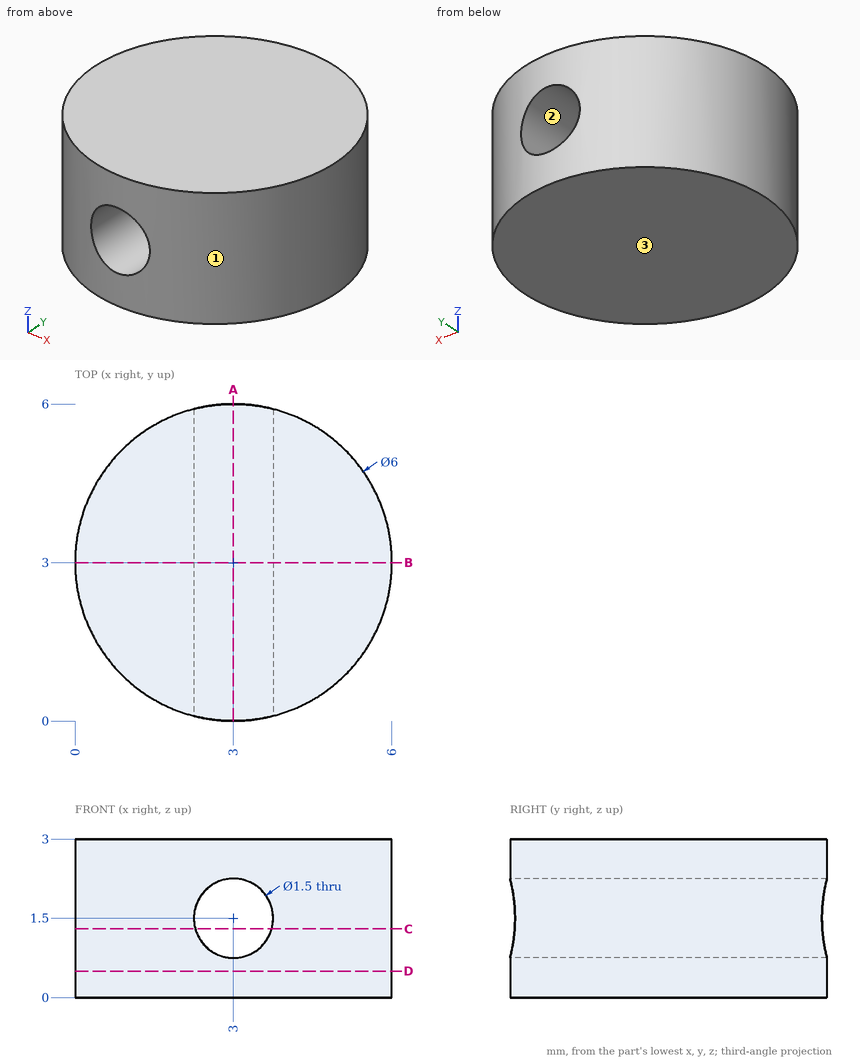
Could you check a few things on this drawing? It's one solid part, dimensions in mm from its lowest x, y, z. Give positions to 0.01 mm unless a question says otherwise; leave off trailing zeros. Order: outer loops, then holes, each group sorted by start corner. A loop starts at its lowest first (then second) coordinate and runs counter-clockwise, first axis right, second up.
1. Suppose I cut it at D-D (z = 0.5). Write out the boundary of the cut face in (x, y), plus the area to 3 significant figures.
Answers below:
outline: circle Ø6 at (3, 3)
area: 28.3 mm2
2. Suppose I cut it at B-B (y = 3). Write out the boundary of the cut face in (x, z).
Answers below:
outline: (0, 0) - (6, 0) - (6, 3) - (0, 3) - close; hole circle Ø1.5 at (3, 1.5)
3. Thinking about a two-plate mould opening in X: for the marked faces 1, 2 and 3, which applies, +X half, -X half, draft (parallel to the pull), parting line (faces both ways), or undercut?
Answers below:
face 1: parting line
face 2: undercut
face 3: draft
4. Suppose I cut it at A-A (x = 3). Write out the boundary of the cut face in (y, z), plus the area to 3 significant figures.
Answers below:
outline: (0, 0) - (6, 0) - (6, 0.75) - (0, 0.75) - close; (0, 2.25) - (6, 2.25) - (6, 3) - (0, 3) - close
area: 9.00 mm2
5. Suppose I cut it at C-C (z = 1.3). Write out the boundary of the cut face in (x, y), plus the area to 3 significant figures.
Answers below:
outline: (2.28, 0.09) - (2.28, 5.91) arc R3 ccw to start; (3.72, 0.09) arc R3 ccw to (3.72, 5.91) - close
area: 19.7 mm2
6. I need wall thicknesses on L1, parallel to Z at x = 3, y = 4.75; L2, parallel to X at y = 0.75, z = 2; L3, parallel to X at y = 1.75, z = 1.95. Which ranges of each line are inside material? Lowest first, please.
Answers below:
L1: z = 0 to 0.75, 2.25 to 3
L2: x = 1.02 to 2.44, 3.56 to 4.98
L3: x = 0.27 to 2.4, 3.6 to 5.73
